Geometry check sheet. Reference: the model listing, model coordinates, mm. Face numbers are marked on the shaded views. A direction names the side the tool comes from. Give positions to 0.01 mm unless a question says otherwise; leave off trailing zeros. Write each loop counter-clockwise with the first axis right and the second up, starting at its lowest first coordinate (ties: lowest second). Pieces come first, ordered by that corner, then holes.
(1) Tool access check on the marked faces 1 and 2. Record the directions out of +Z, -Z, +X, -X, +Y, -Y that give a thin tool (end or side, any length) a straight path to the whole face; none if there is none.
(2) Cross-section at A-A (x = 0). Record the boundary of the cut face in (y, z).
(3) Depth check by flat-ended pin: P1, Ø2, axis at x = 1, z = 0.5, coming from the -Y side; P2, Ø2, axis at x = -7, y = 1.5, coming from the +Z side. Enter the tip coordinate at first touch or a pass-through.
(4) Cross-section at C-C (z = 2.2). Record the boundary of the cut face in (x, y), and give its area (3 significant figures).
(5) Thickness scan on line 1 along Z through (x, y) = (-5.25, 1.5); line 2 along X through (y, z) = (6.75, -0.6); line 3 along X through (y, z) = (1, -0.7). Record the ranges inside material, lowest first.
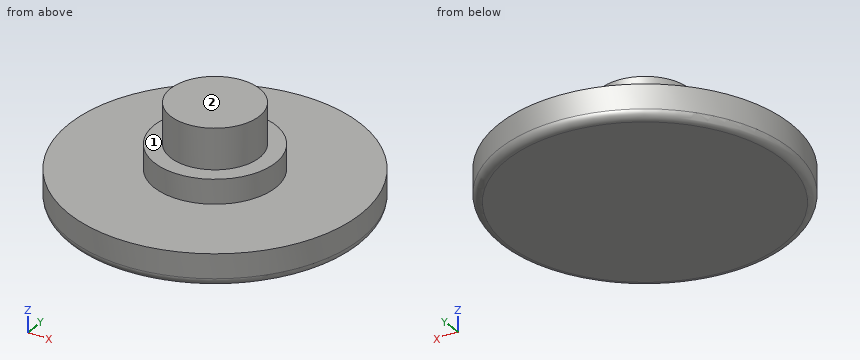
```python
from build123d import *


with BuildPart() as f1:
    # F0 (on Front) → F1 (revolve)
    with BuildSketch(Plane.XZ):
        with BuildLine():
            Line((0, -2), (0, 4))
            Line((0, 4), (-2.75, 4))
            Line((-2.75, 4), (-2.75, 1.5))
            Line((-2.75, 1.5), (-3.75, 1.5))
            Line((-3.75, 1.5), (-3.75, 0))
            Line((-3.75, 0), (-9, 0))
            Line((-9, 0), (-9, -1.5))
            ThreePointArc((-9, -1.5), (-8.853553, -1.853553), (-8.5, -2))
            Line((-8.5, -2), (0, -2))
        make_face()
    revolve(axis=Axis((0, 0, 1), (0, 0, 1)))


solid = f1.part
```
Reply:
1. face 1: +Z
1. face 2: +Z, +X, -X, +Y, -Y
2. outline: (-9, -1.5) arc R0.5 ccw to (-8.5, -2) - (8.5, -2) arc R0.5 ccw to (9, -1.5) - (9, 0) - (3.75, 0) - (3.75, 1.5) - (2.75, 1.5) - (2.75, 4) - (-2.75, 4) - (-2.75, 1.5) - (-3.75, 1.5) - (-3.75, 0) - (-9, 0) - close
3. P1: stops at y = -9
3. P2: stops at z = 0
4. outline: circle Ø5.5 at (0, 0)
4. area: 23.8 mm2
5. line 1: z = -2 to 0
5. line 2: x = -5.95 to 5.95
5. line 3: x = -8.94 to 8.94
